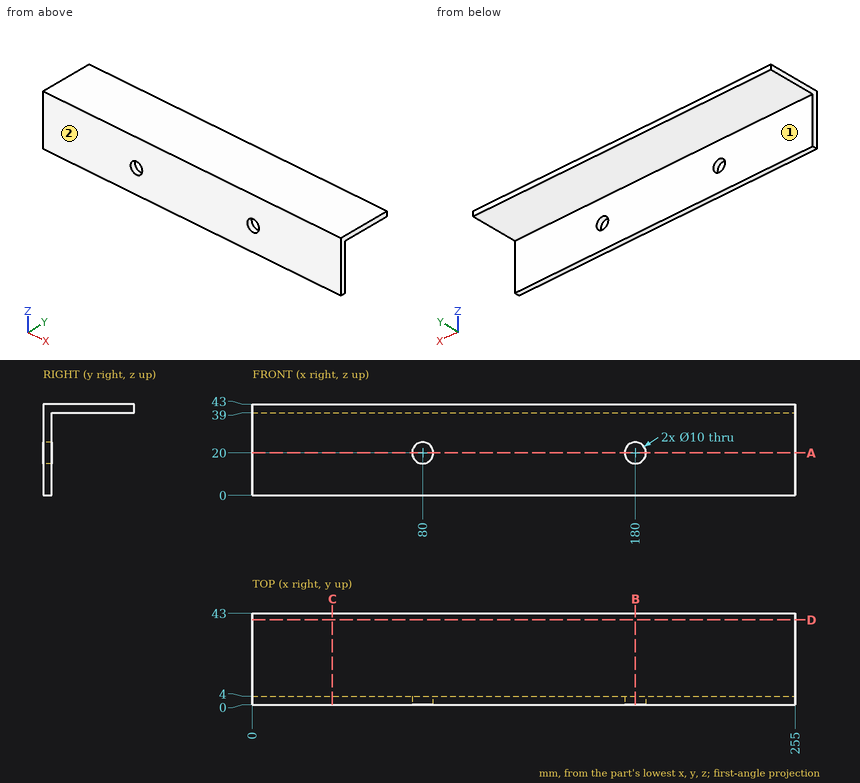
Input: dimensioned drawing with shaded views. Units: mm. Origin: part minimum x, y, z. A direction names the side the tool comes from. Coordinates: 2 decimals unless noted, no trailing zeros. Loops run counter-clockwise (first coordinate to the right, second up) from the corner with the lowest first, then second, coordinate; pieces in that order, holes last. Notation, with made-up numbers: M 63,-11.5 L 80,-11.5 A32 cw 80,27.5 Z; hole C 34,59 d2. An arc over 180 degrees is marked long. Put each result on its own line as item: value.
(1) Cut plane D-D on y = 40. Return the cut outline in (x, z).
Answer sheet:
outline: M 0,39 L 255,39 L 255,43 L 0,43 Z
(2) Cut plane C-C on x = 37.5. Return the cut outline in (y, z).
Answer sheet:
outline: M 0,0 L 4,0 L 4,39 L 43,39 L 43,43 L 0,43 Z
(3) Material intervals for probe 1 along Z at (x, y) = (180, 1); probe 2 along Z at (x, y) = (43, 20.5); probe 3 along Y at (x, z) = (206, 32), sorted ascending.
Answer sheet:
probe 1: z = 0 to 15, 25 to 43
probe 2: z = 39 to 43
probe 3: y = 0 to 4
(4) Access query for the marked faces 1 and 2. Directions: +Z, -Z, +X, -X, +Y, -Y. A direction counts if a zero-diameter tool reaches every point of the face in a straight line with its end or side. Return the directions, or none.
Answer sheet:
face 1: -Z, +X, -X, +Y
face 2: +Z, -Z, +X, -X, -Y
(5) First-contact query: pin 1 (5 mm diameter, centred on x = 31, y = 25, fed in from -Z); pin 2 (3 mm diameter, centred on x = 106.5, z = 6, fed in from -Y); pin 3 (13 mm diameter, centred on x = 80, z = 20, fed in from +Y). Flat tips, straight axial feed; report the tip coordinate or a pass-through.
Answer sheet:
pin 1: stops at z = 39
pin 2: stops at y = 0
pin 3: stops at y = 4
(6) Cut plane A-A on z = 20. Return the cut outline in (x, y), then the cut area to 3 significant figures.
Answer sheet:
outline: M 0,0 L 75,0 L 75,4 L 0,4 Z; M 85,0 L 175,0 L 175,4 L 85,4 Z; M 185,0 L 255,0 L 255,4 L 185,4 Z
area: 940 mm^2
(7) Cut plane B-B on x = 180. Return the cut outline in (y, z), then the cut area to 3 significant figures.
Answer sheet:
outline: M 0,0 L 4,0 L 4,15 L 0,15 Z; M 0,25 L 4,25 L 4,39 L 43,39 L 43,43 L 0,43 Z
area: 288 mm^2
